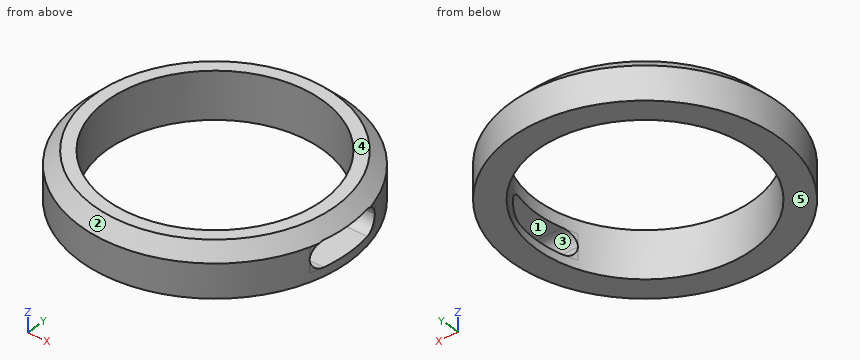
```python
from build123d import *

# Parameters (mm, degrees)
F0_R         = 10
F0_R_2       = 8.05
F1_DEPTH     = 3.5
F3_DEPTH     = 16.9
F4_T4_DEPTH  = 7.0692849199
F4_S5_R      = 10
F4_T6_DEPTH  = 5
F4_S7_R      = 8.05
F4_T8_DEPTH  = 5
F4_T12_DEPTH = 7.0692849199
F4_S13_R     = 10
F4_T14_DEPTH = 5
F4_S15_R     = 8.05
F4_T16_DEPTH = 5
F4_T20_DEPTH = 7.0692849199
F4_S21_R     = 10
F4_T22_DEPTH = 5
F4_S23_R     = 8.05
F4_T24_DEPTH = 5
F4_T28_DEPTH = 7.0692849199
F4_S29_R     = 10
F4_T30_DEPTH = 5
F4_S31_R     = 8.05
F4_T32_DEPTH = 5


# Not quite as in the source:
# - a fillet or chamfer that OpenCascade refuses, or shapes differently, is made with other operations: its cross-section is extruded or revolved along the edge and cut away or added


with BuildPart() as f1:
    # F0 (on Top) → F1 (new body)
    with BuildSketch(Plane.XY):
        Circle(F0_R)
        Circle(F0_R_2, mode=Mode.SUBTRACT)
    extrude(amount=F1_DEPTH)

    # F2 (on Right) → F3 (cut)
    with BuildSketch(Plane.YZ):
        Polygon((3, 0.65), (3, 2.55), (-3, 2.55), (-3, 0.65), (0, 0.65), align=None)
    extrude(amount=F3_DEPTH, mode=Mode.SUBTRACT)

    # F4: fillet of radius 1 on 4 edges, made by hand


with BuildPart() as f4_tool2:
    # F4_s3 → F4_t4 (new body)
    with BuildSketch(Plane.YZ.offset(4.9701070943)):
        with BuildLine():
            ThreePointArc((2, 2.55), (2.7071067812, 2.2571067812), (3, 1.55))
            Line((3, 1.55), (3, 2.55))
            Line((3, 2.55), (2, 2.55))
        make_face()
    extrude(amount=F4_T4_DEPTH)

    # F4_s5 → F4_t6 (intersect, symmetric)
    with BuildSketch(Plane.XY.offset(2)):
        Circle(F4_S5_R)
    extrude(amount=F4_T6_DEPTH, both=True, mode=Mode.INTERSECT)

    # F4_s7 → F4_t8 (cut, symmetric)
    with BuildSketch(Plane.XY.offset(2)):
        Circle(F4_S7_R)
    extrude(amount=F4_T8_DEPTH, both=True, mode=Mode.SUBTRACT)


with BuildPart() as f1_1:
    add(f1.part)

    # F4_t1: union F4_tool2
    add(f4_tool2.part)


with BuildPart() as f4_tool10:
    # F4_s11 → F4_t12 (new body)
    with BuildSketch(Plane.YZ.offset(4.9701070943)):
        with BuildLine():
            ThreePointArc((2, 0.65), (2.7071067812, 0.9428932188), (3, 1.65))
            Line((3, 1.65), (3, 0.65))
            Line((3, 0.65), (2, 0.65))
        make_face()
    extrude(amount=F4_T12_DEPTH)

    # F4_s13 → F4_t14 (intersect, symmetric)
    with BuildSketch(Plane.XY.offset(1.1)):
        Circle(F4_S13_R)
    extrude(amount=F4_T14_DEPTH, both=True, mode=Mode.INTERSECT)

    # F4_s15 → F4_t16 (cut, symmetric)
    with BuildSketch(Plane.XY.offset(1.1)):
        Circle(F4_S15_R)
    extrude(amount=F4_T16_DEPTH, both=True, mode=Mode.SUBTRACT)


with BuildPart() as f1_2:
    add(f1_1.part)

    # F4_t9: union F4_tool10
    add(f4_tool10.part)


with BuildPart() as f4_tool18:
    # F4_s19 → F4_t20 (new body)
    with BuildSketch(Plane.YZ.offset(4.9701070943)):
        with BuildLine():
            ThreePointArc((-3, 1.55), (-2.7071067812, 2.2571067812), (-2, 2.55))
            Line((-2, 2.55), (-3, 2.55))
            Line((-3, 2.55), (-3, 1.55))
        make_face()
    extrude(amount=F4_T20_DEPTH)

    # F4_s21 → F4_t22 (intersect, symmetric)
    with BuildSketch(Plane.XY.offset(2)):
        Circle(F4_S21_R)
    extrude(amount=F4_T22_DEPTH, both=True, mode=Mode.INTERSECT)

    # F4_s23 → F4_t24 (cut, symmetric)
    with BuildSketch(Plane.XY.offset(2)):
        Circle(F4_S23_R)
    extrude(amount=F4_T24_DEPTH, both=True, mode=Mode.SUBTRACT)


with BuildPart() as f1_3:
    add(f1_2.part)

    # F4_t17: union F4_tool18
    add(f4_tool18.part)


with BuildPart() as f4_tool26:
    # F4_s27 → F4_t28 (new body)
    with BuildSketch(Plane.YZ.offset(4.9701070943)):
        with BuildLine():
            ThreePointArc((-2, 0.65), (-2.7071067812, 0.9428932188), (-3, 1.65))
            Line((-3, 1.65), (-3, 0.65))
            Line((-3, 0.65), (-2, 0.65))
        make_face()
    extrude(amount=F4_T28_DEPTH)

    # F4_s29 → F4_t30 (intersect, symmetric)
    with BuildSketch(Plane.XY.offset(1.1)):
        Circle(F4_S29_R)
    extrude(amount=F4_T30_DEPTH, both=True, mode=Mode.INTERSECT)

    # F4_s31 → F4_t32 (cut, symmetric)
    with BuildSketch(Plane.XY.offset(1.1)):
        Circle(F4_S31_R)
    extrude(amount=F4_T32_DEPTH, both=True, mode=Mode.SUBTRACT)


with BuildPart() as f1_4:
    add(f1_3.part)

    # F4_t25: union F4_tool26
    add(f4_tool26.part)

    # F5: chamfer of 1 on 1 edges, made by hand

    # F5_s1 → F5_t2 (revolve, cut)
    with BuildSketch(Plane.XZ):
        Polygon((10, 2.5), (9, 3.5), (10, 3.5), align=None)
    revolve(axis=Axis((0, 0, 3.5), (0, 0, 1)), mode=Mode.SUBTRACT)


solid = f1_4.part
```
For this review, take the finished solid that the model builds, in its own axes (mm). Face numbers are marked on the shaded views. A direction names the side the tool comes from. Round coordinates to 2 decimals unless told otherwise and drop trailing zeros. Order: outer loops, then holes, each group sorted by start corner. A loop starts at its lowest first (then second) coordinate and runs counter-clockwise, first axis right, second up.
Q1. We need section C-C, the plane z = 3. Give the boundary of the cut face in (x, y).
Findings below:
outline: circle Ø19 at (0, 0); hole circle Ø16.1 at (0, 0)
Q2. Machinability: for the marked faces 1 and 2, which of the approach directions +Z, -Z, +X, -X, +Y, -Y give a long, thin tool a straight path to every point of the face, cutting with its end or side? Answer none if there is none.
Findings below:
face 1: +X
face 2: +Z
Q3. Insertion check: P1, Ø4, axis at x = -5.5, y = -1, coming from the +Z side; P2, Ø2, axis at y = 5.5, z = 2, coming from the -X side; P3, Ø1, axis at y = 7, z = 1.5, coming from the +X side. Each pin has a flat end and moves straight along its axis. Give the tip position at first contact, or say it passes through.
Findings below:
P1: passes through
P2: stops at x = -8.93
P3: stops at x = 7.6
Q4. Wall thickness on line 1 (Y direction, x = 0, z = 0.95); line 2 (Y direction, x = 3.5, z = 0.55); line 3 (X direction, y = 2.75, z = 2.75): over which ranges is each line inside the solid? List them lowest first.
Findings below:
line 1: y = -10 to -8.05, 8.05 to 10
line 2: y = -9.37 to -7.25, 7.25 to 9.37
line 3: x = -9.35 to -7.57, 7.57 to 9.35
Q5. Mouldability with a two-part tool opening along Z and no side actions: class the marked faces 3, 4 and 5 as pulls with the +Z half, pulls with the -Z half, needs draft (parallel to the pull), parting line crosses it, or undercut.
Findings below:
face 3: undercut
face 4: pulls with the +Z half
face 5: pulls with the -Z half
Q6. We need section A-A, the plane y = 0. Give the boundary of the cut face in (x, z).
Findings below:
outline: (-10, 0) - (-8.05, 0) - (-8.05, 3.5) - (-9, 3.5) - (-10, 2.5) - close; (8.05, 0) - (10, 0) - (10, 0.65) - (8.05, 0.65) - close; (8.05, 2.55) - (9.95, 2.55) - (9, 3.5) - (8.05, 3.5) - close
Q7. We need section D-D, the plane z = 1.25. Give the boundary of the cut face in (x, y).
Findings below:
outline: (7.5, -2.92) arc R8.05 cw (long way) to (7.5, 2.92) - (9.57, 2.92) arc R10 ccw (long way) to (9.57, -2.92) - close
Q8. We need section B-B, the plane x = 0. Give the boundary of the cut face in (y, z), plus the area to 4 significant figures.
Findings below:
outline: (-10, 0) - (-8.05, 0) - (-8.05, 3.5) - (-9, 3.5) - (-10, 2.5) - close; (8.05, 0) - (10, 0) - (10, 2.5) - (9, 3.5) - (8.05, 3.5) - close
area: 12.65 mm2
